from build123d import *

# Parameters (mm, degrees)
F1_DEPTH = 3.81
F2_W     = 23.2185392497
F2_H     = 19.05
F3_DEPTH = 25.4
F4_R     = 5.08


with BuildPart() as f1:
    # F0 (on Top) → F1 (new body)
    with BuildSketch(Plane.XY):
        with BuildLine():
            Line((18.5659871323, 88.1776532905), (-32.2340128677, 88.1776532905))
            Line((-32.2340128677, 88.1776532905), (-32.2340128677, -64.2223467095))
            Line((-32.2340128677, -64.2223467095), (-5.5640128677, -64.2223467095))
            Line((-5.5640128677, -64.2223467095), (-5.5640128677, -38.8223467095))
            Line((-5.5640128677, -38.8223467095), (-5.9028261468, -38.8223467095))
            ThreePointArc((-5.9028261468, -38.8223467095), (-15.4278261468, -29.2973467095), (-5.9028261468, -19.7723467095))
            Line((-5.9028261468, -19.7723467095), (-5.5640128677, -19.7723467095))
            Line((-5.5640128677, -19.7723467095), (-5.5640128677, 19.5976532905))
            Line((-5.5640128677, 19.5976532905), (18.5659871323, 19.5976532905))
            Line((18.5659871323, 19.5976532905), (18.5659871323, 88.1776532905))
        make_face()
        with BuildLine():
            ThreePointArc((-7.4690128677, 43.7276532905), (-16.9940128677, 53.2526532905), (-7.4690128677, 62.7776532905))
            Line((-7.4690128677, 62.7776532905), (1.4209871323, 62.7776532905))
            ThreePointArc((1.4209871323, 62.7776532905), (10.9459871323, 53.2526532905), (1.4209871323, 43.7276532905))
            Line((1.4209871323, 43.7276532905), (-7.4690128677, 43.7276532905))
        make_face(mode=Mode.SUBTRACT)
    extrude(amount=F1_DEPTH)

    # F2 (on face) → F3 (cut)
    with BuildSketch(Plane.XY.offset(3.81)):
        with Locations((13.0302567572, 53.2526532905)):
            Rectangle(F2_W, F2_H)
    extrude(amount=-F3_DEPTH, mode=Mode.SUBTRACT)

    # F4
    f4_edges = [f1.edges().sort_by_distance(p)[0] for p in [
        (18.565987, 88.177653, 1.905),
        (-32.234013, 88.177653, 1.905),
        (-32.234013, -64.222347, 1.905),
        (-5.564013, -64.222347, 1.905),
        (-5.564013, -19.772347, 1.905),
        (-5.564013, -38.822347, 1.905),
        (18.565987, 19.597653, 1.905),
        (-5.564013, 19.597653, 1.905),
        (18.565987, 43.727653, 1.905),
        (18.565987, 62.777653, 1.905),
    ]]
    fillet(f4_edges, radius=F4_R)


solid = f1.part
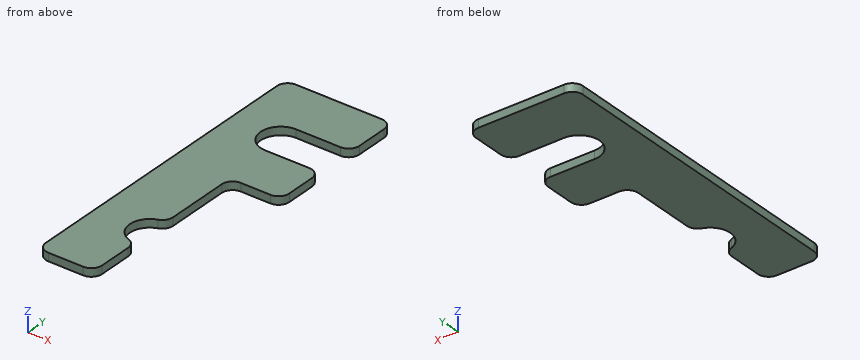
Could you check a few things on this model? Use its own coordinates, in mm. Give positions to 0.01 mm unless a question says otherwise; leave off trailing zeros. Order: outer loops, then holes, each group sorted by start corner. A loop starts at its lowest first (then second) coordinate and runs counter-clockwise, first axis right, second up.
1. Suppose I cut it at A-A (x = 3). List the corners of the cut face in (y, z) for me.
2. Suppose I cut it at B-B (x = -13.5). List the corners of the cut face in (y, z) for me.
3. Suppose I cut it at C-C (y = -14). List the corners of the cut face in (x, z) for me.
4. I need wall thicknesses on L1, parallel to Y at x = -8, z = 0.95; L2, parallel to Y at x = 5, z = 1.75; L3, parallel to Y at x = -12, z = 3. Which ranges of each line are inside material? Lowest first, please.
5. Will these pins go through, and if not, where does the flat tip stop? P1, Ø1.1, axis at y = -3.5, z = 2.5, coming from the +X side; P2, Ø1.9, axis at x = 3, z = 1.5, coming from the -Y side.
6. Suppose I cut it at D-D (x = -4). List the corners of the cut face in (y, z) for me, plus the area to 3 significant figures.
Solved:
1. outline: (19.6, 0) - (43.73, 0) - (43.73, 3.81) - (19.6, 3.81) - close; (62.78, 0) - (88.18, 0) - (88.18, 3.81) - (62.78, 3.81) - close
2. outline: (-64.22, 0) - (-35.04, 0) - (-35.04, 3.81) - (-64.22, 3.81) - close; (-23.55, 0) - (45.88, 0) - (45.88, 3.81) - (-23.55, 3.81) - close; (60.63, 0) - (88.18, 0) - (88.18, 3.81) - (60.63, 3.81) - close
3. outline: (-32.23, 0) - (-5.56, 0) - (-5.56, 3.81) - (-32.23, 3.81) - close
4. L1: y = -63.48 to -38.77, -19.82 to 43.74, 62.76 to 88.18
4. L2: y = 19.6 to 43.73, 62.78 to 88.18
4. L3: y = -64.22 to -36.62, -21.98 to 44.87, 61.63 to 88.18
5. P1: stops at x = -5.56
5. P2: stops at y = 19.6
6. outline: (18.18, 0) - (43.73, 0) - (43.73, 3.81) - (18.18, 3.81) - close; (62.78, 0) - (88.18, 0) - (88.18, 3.81) - (62.78, 3.81) - close
6. area: 194 mm2
